For this review, take the finished solid that the model builds, in its own axes (mm). Face numbers are marked on the shaded views. A direction names the side the tool comes from. Give positions to 0.01 mm unless a question says otherwise; leave off trailing zeros. Loops run counter-clockwise (first coordinate to the right, second up) from the corner with the lowest first, then second, coordinate; pieces in that order, holes last. Notation, with made-up numbers: (-23, 15) - (10, 15) arc R25 ccw to (10, 46) - close; hole circle Ø10 at (74, -31.75). An arc over 180 degrees is marked (long way). Answer in a Markdown table with one row per item.
Solid Edge part; units mm, degrees
sketch "Sketch1" plane through (0, 0, 0) normal (0, 0, 1) x (1, 0, 0)
  line L0 (-2.0207, 3.5) -> (2.0207, 3.5)
  line L1 (2.0207, 3.5) -> (4.0415, 0)
  line L2 (4.0415, 0) -> (2.0207, -3.5)
  line L3 (2.0207, -3.5) -> (-2.0207, -3.5)
  line L4 (-2.0207, -3.5) -> (-4.0415, 0)
  line L5 (-4.0415, 0) -> (-2.0207, 3.5)
extrude "Protrusion1" add sketch "Sketch1" along normal blind 4.65
sketch "Sketch2" plane through (0, 0, 0) normal (0, -1, 0) x (1, 0, 0)
  line L0 (4.0415, 3.85) -> (2.574, 5.3174)
  line L1 (2.574, 5.3174) -> (4.6962, 5.3174)
  line L2 (4.6962, 5.3174) -> (4.6962, 3.85)
  line L3 (4.6962, 3.85) -> (4.0415, 3.85)
revolve "RevolvedCutout1" cut sketch "Sketch2" angle 360 about axis through (0, 0, 54) along (0, 0, -1)
sketch "Sketch3" plane through (0, 0, 0) normal (0, -1, 0) x (1, 0, 0)
  line L0 (0, 0) -> (5, 0)
  line L1 (5, 0) -> (5, 0.5)
  line L2 (5, 0.5) -> (2.7639, 2.7361)
  line L3 (2.7639, 2.7361) -> (0, 2.7361)
  line L4 (0, 2.7361) -> (0, 0)
  dimension "D1" = 5
revolve "RevolvedProtrusion1" add sketch "Sketch3" angle 360 about axis through (0, 0, 54) along (0, 0, -1)
fillet "Verrundung_1" radius 0.2 2 edges at (-5, 0, 0.5) (-5, 0, 0)
hole "Bohrung_1" at (0, 0, 4.65) direction (0, 0, -1) diameter 4 end through all
chamfer "Fase_1" distance 0.3 angle 45 2 edges at (0, 2, 4.65) (2, 0, 0)
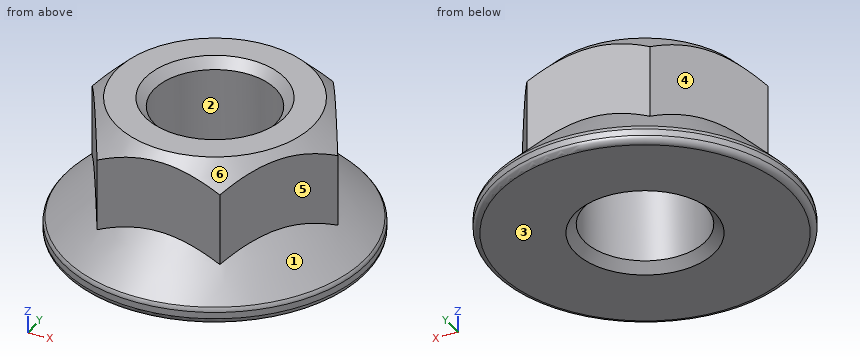
1. We need section A-A, the plane z = 2.55. Give the boundary of the cut face in (x, y), and give its area (3 significant figures).
Values:
| item | result |
|---|---|
| outline | (-4.04, 0) - (-2.02, -3.5) - (2.02, -3.5) - (4.04, 0) - (2.02, 3.5) - (-2.02, 3.5) - close; hole circle Ø4 at (0, 0) |
| area | 29.9 mm^2 |
2. Mouldability with a two-part tool opening along X and no side actions: class the marked faces 1, 2 and 3 as released by +X, released by -X, zero draft, split by the parting line, or undercut.
Values:
| item | result |
|---|---|
| face 1 | split by the parting line |
| face 2 | undercut |
| face 3 | zero draft |
3. Clearance check with flat-ended pins moving along their axes: pin 1 (2 mm diameter, centred on x = -2.5, z = 2, fed in from +Y); pin 2 (2.5 mm diameter, centred on x = 0, z = 2.5, fed in from +Y); pin 3 (1.5 mm diameter, centred on x = 0, z = 2.5, fed in from -Y). State where each tip first meets the part, or that it passes through.
Values:
| item | result |
|---|---|
| pin 1 | stops at y = 3.89 |
| pin 2 | stops at y = 4.25 |
| pin 3 | stops at y = -3.75 |
4. We need section B-B, the plane z = 1.7. Give the boundary of the cut face in (x, y).
Values:
| item | result |
|---|---|
| outline | (-4.04, 0) - (-3.77, -0.47) arc R3.8 ccw to (-2.29, -3.03) - (-2.02, -3.5) - (-1.48, -3.5) arc R3.8 ccw to (1.48, -3.5) - (2.02, -3.5) - (2.29, -3.03) arc R3.8 ccw to (3.77, -0.47) - (4.04, 0) - (3.77, 0.47) arc R3.8 ccw to (2.29, 3.03) - (2.02, 3.5) - (1.48, 3.5) arc R3.8 ccw to (-1.48, 3.5) - (-2.02, 3.5) - (-2.29, 3.03) arc R3.8 ccw to (-3.77, 0.47) - close; hole circle Ø4 at (0, 0) |
5. For the marked faces 4, 5 and 6, list the 3-axis set-ups (+Z, -Z, +X, -X, +Y, -Y) from which the entire face can be reached by the end or side of a thin tool; tool diameter is ignored.
Values:
| item | result |
|---|---|
| face 4 | +Z, -X, +Y |
| face 5 | +Z, +X, -Y |
| face 6 | +Z |
6. We need section C-C, the plane z = 4. Give the boundary of the cut face in (x, y), and give its area (3 significant figures).
Values:
| item | result |
|---|---|
| outline | (-3.88, -0.28) - (-2.18, -3.22) arc R3.89 ccw to (-1.7, -3.5) - (1.7, -3.5) arc R3.89 ccw to (2.18, -3.22) - (3.88, -0.28) arc R3.89 ccw to (3.88, 0.28) - (2.18, 3.22) arc R3.89 ccw to (1.7, 3.5) - (-1.7, 3.5) arc R3.89 ccw to (-2.18, 3.22) - (-3.88, 0.28) arc R3.89 ccw to start; hole circle Ø4 at (0, 0) |
| area | 29.6 mm^2 |
7. Wall thickness on line 1 (Y direction, x = 0, z = 2.55); line 2 (Y direction, x = 1, z = 0.35); line 3 (X direction, y = 1.5, z = 3.8): over which ranges is each line inside the solid? List them lowest first. Write a range as [from, to].
Values:
| item | result |
|---|---|
| line 1 | y = [-3.5, -2], [2, 3.5] |
| line 2 | y = [-4.9, -1.73], [1.73, 4.9] |
| line 3 | x = [-3.18, -1.32], [1.32, 3.18] |
